Model file for the job. Use its own axes, mm. A direction names the side the tool comes from. Give positions to 0.01 mm unless a question says otherwise; leave off trailing zeros. Write each loop counter-clockwise with the first axis right and the second up, starting at its lowest first coordinate (ties: lowest second). Pieces come first, ordered by that corner, then holes. Notation, with made-up numbers: (72, 84) - (130, 84) arc R35 ccw to (130, 118) - close; hole circle Ø7 at (31.25, -36.5). An arc over 180 degrees is marked (long way). One line per item, written item: value. Start each with the question number.
(1) Probe L1, parallel to Z at x = 0, y = 7.5; L2, parallel to Z at x = 0, y = -13; L3, parallel to Y at x = 8.5, z = 22. List the from-to ranges inside material, lowest first.
(2) Cut at B-B, the plane x = 0. List the corners of the cut face in (y, z).
(3) Cut at C-C, the plane y = 19. List the corners of the cut face in (x, z).
(4) Cut at D-D, the plane y = 4.5. List the corners of the cut face in (x, z), and give its area (3 significant figures).
(5) 3-axis set-ups, long thin cutter, end or side, ignore diameter. For faces 1 (the face through (23.846, -14.965, 7.509)), 2 (the face through (47.69, -0.18, 15.02)), 3 (the face through (23.846, 15.035, 7.509)): which of +Z, -Z, +X, -X, +Y, -Y reach the whole face in a straight line?
(6) Cut at A-A, the plane z = 0. List the corners of the cut face in (x, y).
(7) Mould opens along X. For faces 4 (the face through (6, 22.5, 30)), 5 (the face through (-3.286, 17.743, 25.028)), 6 (the face through (-32.128, 22.014, -24.635)) say: pulls with the +X half, pulls with the -X half, needs draft (parallel to the pull), parting line crosses it, or undercut.
(8) Drop flat-ended pins along their axis: P1, Ø5, axis at x = -27.5, y = -10, coming from the +Z side; P2, Ø3, axis at y = 1.5, z = 10.5, coming from the +X side; P3, Ø10, axis at x = -17.5, z = -4.5, coming from the -Y side; P4, Ø5, axis at y = 1.5, z = 1.5, coming from the -X side. Give the stop position or say it passes through.
from build123d import *

# Parameters (mm, degrees)
F0_R     = 50
F0_R_2   = 25
F1_DEPTH = 22.5
F0_R_3   = 7.5
F2_DEPTH = 12.5
F3_SIZE  = 10
F4_SIZE  = 5


with BuildPart() as f1:
    # F0 (on Front) → F1 (new body, symmetric)
    with BuildSketch(Plane.XZ):
        Circle(F0_R)
        Circle(F0_R_2, mode=Mode.SUBTRACT)
    extrude(amount=F1_DEPTH, both=True)

    # F0 (on Front) → F2 (join, symmetric)
    with BuildSketch(Plane.XZ):
        Circle(F0_R_2)
        Circle(F0_R_3, mode=Mode.SUBTRACT)
    extrude(amount=F2_DEPTH, both=True)

    # F3
    f3_edges = [f1.edges().sort_by_distance(p)[0] for p in [
        (-50, -22.5, 0),
        (-50, 22.5, 0),
    ]]
    chamfer(f3_edges, length=F3_SIZE)

    # F4
    f4_edges = [f1.edges().sort_by_distance(p)[0] for p in [
        (-25, -22.5, 0),
        (-25, 22.5, 0),
    ]]
    chamfer(f4_edges, length=F4_SIZE)


solid = f1.part
Answers follow:
1. L1: z = -50 to -7.5, 7.5 to 50
1. L2: z = -49.5 to -25, 25 to 49.5
1. L3: y = -12.5 to 12.5
2. outline: (-22.5, -40) - (-12.5, -50) - (12.5, -50) - (22.5, -40) - (22.5, -30) - (17.5, -25) - (12.5, -25) - (12.5, -7.5) - (-12.5, -7.5) - (-12.5, -25) - (-17.5, -25) - (-22.5, -30) - close; (-22.5, 30) - (-17.5, 25) - (-12.5, 25) - (-12.5, 7.5) - (12.5, 7.5) - (12.5, 25) - (17.5, 25) - (22.5, 30) - (22.5, 40) - (12.5, 50) - (-12.5, 50) - (-22.5, 40) - close
3. outline: circle Ø87 at (0, 0); hole circle Ø53 at (0, 0)
4. outline: circle Ø100 at (0, 0); hole circle Ø15 at (0, 0)
4. area: 7,680 mm²
5. face 1: -Y
5. face 2: +Y, -Y
5. face 3: +Y
6. outline: (-50, -12.5) - (-40, -22.5) - (-30, -22.5) - (-25, -17.5) - (-25, -12.5) - (-7.5, -12.5) - (-7.5, 12.5) - (-25, 12.5) - (-25, 17.5) - (-30, 22.5) - (-40, 22.5) - (-50, 12.5) - close; (7.5, -12.5) - (25, -12.5) - (25, -17.5) - (30, -22.5) - (40, -22.5) - (50, -12.5) - (50, 12.5) - (40, 22.5) - (30, 22.5) - (25, 17.5) - (25, 12.5) - (7.5, 12.5) - close
7. face 4: needs draft
7. face 5: undercut
7. face 6: parting line crosses it
8. P1: stops at z = 43.3
8. P2: stops at x = 49.18
8. P3: stops at y = -12.5
8. P4: stops at x = -50
